Can you work these out from the drawing? Everything is in mm from the part's minimum corner. A direction names the side the tool comes from. Give positions to 0.01 mm unless a question says otherwise; leave off trailing zeros. Loops run counter-clockwise (first coordinate to the right, second up) from the corner with the lowest first, then second, coordinate; pieces in that order, holes last. Notation, with made-up numbers: (53, -13) - (98, -13) arc R13 ccw to (98, -9) - close; hole circle Ø5 at (1.25, 52.5). An arc over 180 degrees is marked (long way). Write each question's results on one line, items separated by ' | '. Start each with the question number.
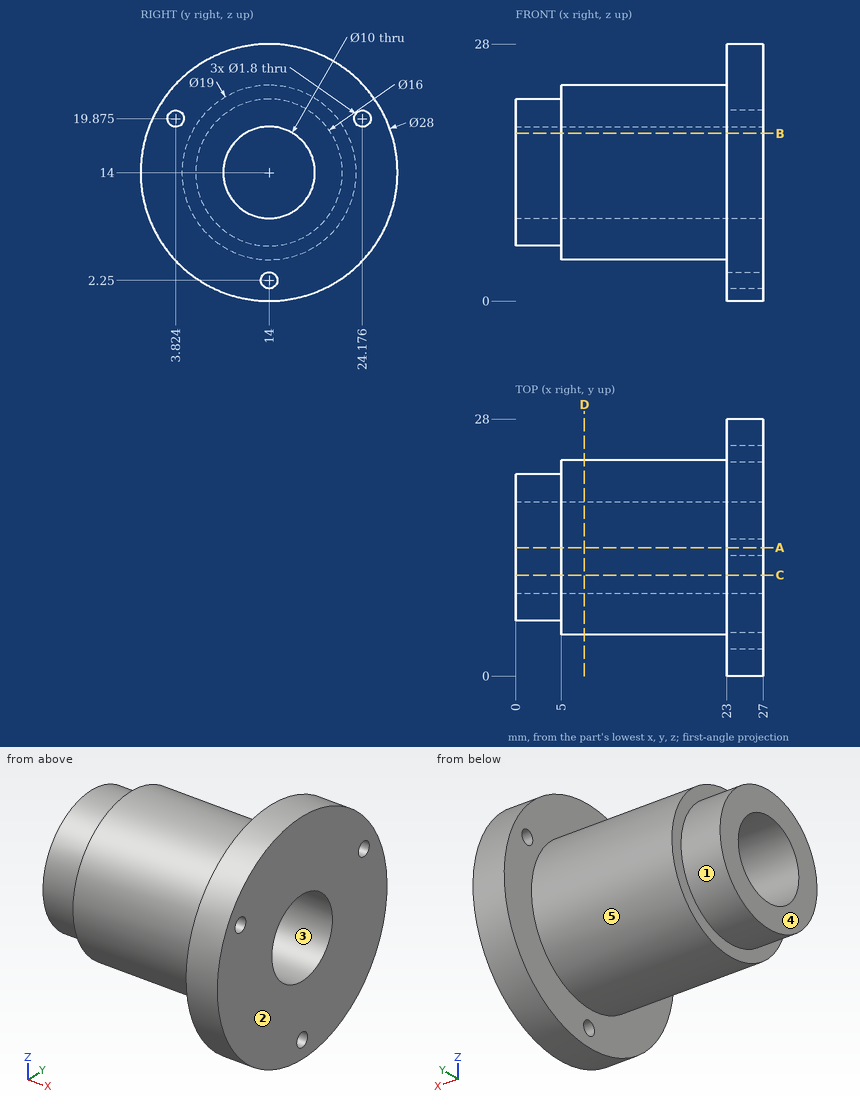
Q1. Which directions (+Z, -Z, +X, -X, +Y, -Y) give clear straight access to the entire face, cutting with the end or side of a thin tool? Please do the marked faces 1 and 2.
Q2. I'm going to push flat-ended pins straight in: pin 1 Ø1 at (y, z) = (5, 20.5) entering from -X; pin 2 Ø4 at (x, z) = (7.5, 13.5) entering from -Y; pin 3 Ø1.5 at (x, y) = (18, 17) entering from +Z. Where does each tip first touch, or does it pass through?
Q3. I want a section at A-A, the plane y = 14. List the corners of the cut face in (x, z) for me, then the cut area to 3 significant figures.
Q4. I want a section at B-B, the plane z = 18.25. List the corners of the cut face in (x, y) for me.
Q5. If we mould it in two halves opening along Y, with no side actions, what happens to the marked faces 3, 4 and 5? For each: +Y half, -Y half, draft (parallel to the pull), parting line (faces both ways), or undercut.
Q6. I want a section at D-D, the plane x = 7.5. List the corners of the cut face in (y, z) for me, then the cut area to 3 significant figures.
Q7. I need wall thicknesses on L1, parallel to Z at x = 24, y = 14.25 (1 decimal); L2, parallel to X at y = 22.75, z = 6; L3, parallel to Z at x = 10.5, y = 10.25. Which ranges of each line are inside material? Lowest first, please. Write a range as from..to.
Q8. I want a section at C-C, the plane y = 11. List the corners of the cut face in (x, z) for me (1 decimal).
Conclusion:
1) face 1: -X | face 2: +Z, -Z, +X, +Y, -Y
2) pin 1: x = 23 | pin 2: y = 4.5 | pin 3: z = 23.23
3) outline: (0, 6) - (5, 6) - (5, 4.5) - (23, 4.5) - (23, 3.15) - (27, 3.15) - (27, 9) - (0, 9) - close; (0, 19) - (27, 19) - (27, 28) - (23, 28) - (23, 23.5) - (5, 23.5) - (5, 22) - (0, 22) - close; (23, 0) - (27, 0) - (27, 1.35) - (23, 1.35) - close | area: 257 mm^2
4) outline: (0, 7.22) - (5, 7.22) - (5, 5.5) - (23, 5.5) - (23, 0.66) - (27, 0.66) - (27, 11.37) - (0, 11.37) - close; (0, 16.63) - (27, 16.63) - (27, 27.34) - (23, 27.34) - (23, 22.5) - (5, 22.5) - (5, 20.78) - (0, 20.78) - close
5) face 3: undercut | face 4: draft | face 5: parting line
6) outline: circle Ø19 at (14, 14); hole circle Ø10 at (14, 14) | area: 205 mm^2
7) L1: 0..1.4, 3.1..9, 19..28 | L2: 23..27 | L3: 5.27..10.69, 17.31..22.73
8) outline: (0, 6.6) - (5, 6.6) - (5, 5) - (23, 5) - (23, 0.3) - (27, 0.3) - (27, 10) - (0, 10) - close; (0, 18) - (27, 18) - (27, 27.7) - (23, 27.7) - (23, 23) - (5, 23) - (5, 21.4) - (0, 21.4) - close
